from build123d import *

# Parameters (mm, degrees)
SKETCH2_W                   = 53.975
SKETCH2_H                   = 19.05
BOSS_EXTRUDE1_DEPTH         = 19.05
F_1_4_0_25_DIAMETER_HOLE1_D = 6.35


with BuildPart() as part:
    # Sketch2 → Boss-Extrude1 (new body)
    with BuildSketch(Plane.XY):
        with Locations((210.84694204, -3.175)):
            Rectangle(SKETCH2_W, SKETCH2_H)
    extrude(amount=BOSS_EXTRUDE1_DEPTH)

    # 1/4 (0.25) Diameter Hole1 (through all)
    with Locations(Plane(origin=(0, 6.35, 0), x_dir=(1, 0, 0), z_dir=(0, 1, 0))):
        with Locations((203.133359856, -10.795)):
            Hole(F_1_4_0_25_DIAMETER_HOLE1_D / 2)

    # Sketch10 → #10 Clearance Hole1 (revolve, cut)
    with BuildSketch(Plane(origin=(230.602380141, 6.35, 9.525), x_dir=(0, 0, 1), z_dir=(1, 0, 0))):
        Polygon((0, 0), (0, 19.05), (5.2197, 19.05), (2.4892, 15.908919064), (2.4892, 0), align=None)
    revolve(axis=Axis((230.602380141, 12.7, 9.525), (0, -1, 0)), mode=Mode.SUBTRACT)


solid = part.part
Could you check a few things on this model? Use its own coordinates, in mm. Give positions to 0.01 mm unless a question says otherwise; leave off trailing zeros. Order: outer loops, then holes, each group sorted by start corner. A loop starts at its lowest first (then second) coordinate and runs counter-clockwise, first axis right, second up.
Item 1: I'm going to push a flat-ended pin straight in: pin 1 (3 mm diameter, centred on x = 230.6, z = 9.52, fed in from +Y). Where does the tip first touch, or does it pass through?
Item 2: If we mould it in two halves opening along X, with no side actions, what happens to faces 1 (the face through (232.811, -1.493, 10.674)), 2 (the face through (206.305, -3.308, 10.655)), 3 (the face through (183.859, -3, 9)), 4 (the face through (210, -3, 0))? For each: pulls with the +X half, pulls with the -X half, needs draft (parallel to the pull), parting line crosses it, or undercut.
Item 3: If we section it at A-A, the plane x = 204: Write out the boundary of the cut face in (y, z).
Item 4: If we section it at B-B, the plane y = -1: Write out the boundary of the cut face in (x, z) (3 decimals), plus the area to 3 significant figures.
Item 5: If we section it at C-C, the plane z = 8.5: Count the separate pieces of the cut face and the enclosed holes in it, plus the area to 3 significant figures.
Item 6: I need wall thicknesses on line 1 (X direction, y = 1.75, z = 10.25); line 2 (X direction, y = -2.5, z = 9.5); line 3 (Z direction, x = 203, y = -4.5). Which ranges of each line are inside material? Lowest first, please.
Values:
1. pin 1: passes through
2. face 1: undercut
2. face 2: undercut
2. face 3: pulls with the -X half
2. face 4: needs draft
3. outline: (-12.7, 0) - (6.35, 0) - (6.35, 7.74) - (-12.7, 7.74) - close; (-12.7, 13.85) - (6.35, 13.85) - (6.35, 19.05) - (-12.7, 19.05) - close
4. outline: (183.859, 0) - (237.834, 0) - (237.834, 19.05) - (183.859, 19.05) - close; hole circle Ø6.35 at (203.133, 10.795); hole circle Ø4.978 at (230.602, 9.525)
4. area: 977 mm2
5. separate pieces: 3
5. enclosed holes: 0
5. area: 849 mm2
6. line 1: x = 183.86 to 200.01, 206.26 to 228.22, 232.98 to 237.83
6. line 2: x = 183.86 to 200.23, 206.03 to 228.11, 233.09 to 237.83
6. line 3: z = 0 to 7.62, 13.97 to 19.05
